Job drawing, mm, ordinate dimensions from the low corner. One solid piece. Give positions to 0.01 mm unless a question says otherwise; leave off trailing zeros. Write each loop counter-clockwise with the first axis right and the second up, starting at its lowest first coordinate (ties: lowest second). Pieces come first, ordered by that corner, then holes. Notation, with made-up numbers: (37.5, -37.5) -> (84.5, -37.5) arc R5 cw to (84.5, -33.5) -> close; hole circle Ø10 at (60, -25). An arc over 180 degrees is marked (long way). Put each result on its own line as item: value. Start each with the question number.
Item 1: Slice it at C-C, the plane x = 88.5. List the corners of the cut face in (y, z), plus the area to 3 significant figures.
Item 2: Slice it at D-D, the plane x = 28. List the corners of the cut face in (y, z).
Item 3: Flat gauge pins, fed straight in: pin 1 Ø12 at (x, y) = (73.5, 218.5) entering from -Z; pin 2 Ø1 at (x, z) = (108, 1.5) entering from +Y; pin 3 Ø1.9 at (x, z) = (35.5, 4) entering from +Y; pin 4 Ø1.5 at (x, z) = (106, 2.5) entering from +Y. Where does each tip first touch, or does it go through?
Item 4: Drill centre lines: line 1 along X through (y, z) = (66.5, 5) (1 decimal); line 2 along Y through (x, z) = (91.5, 5.75); line 3 along Y through (x, z) = (24.5, 4.25). Where is each one in solid material? Low to high.
Item 5: Slice it at A-A, the plane y = 142.5. Give the number of separate pieces and of enclosed holes in the cut face, plus the area to 3 significant figures.
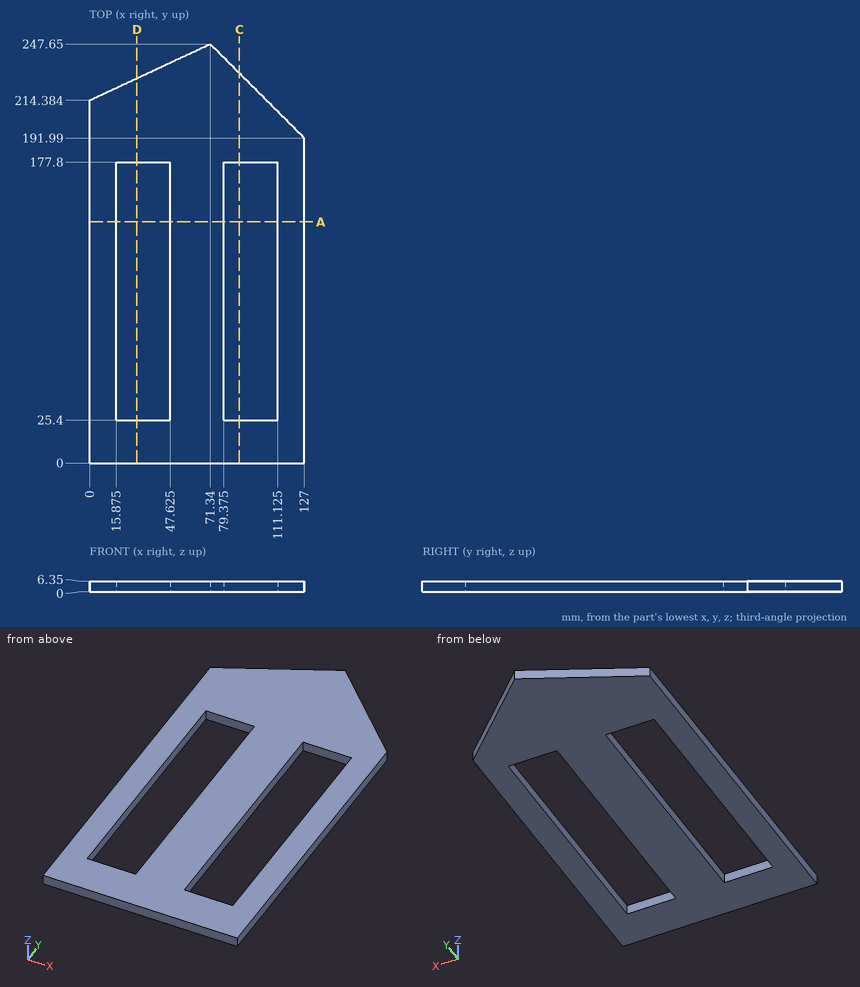
Values follow:
1. outline: (0, 0) -> (25.4, 0) -> (25.4, 6.35) -> (0, 6.35) -> close; (177.8, 0) -> (230.49, 0) -> (230.49, 6.35) -> (177.8, 6.35) -> close
1. area: 496 mm2
2. outline: (0, 0) -> (25.4, 0) -> (25.4, 6.35) -> (0, 6.35) -> close; (177.8, 0) -> (227.44, 0) -> (227.44, 6.35) -> (177.8, 6.35) -> close
3. pin 1: z = 0
3. pin 2: y = 211.49
3. pin 3: y = 231.38
3. pin 4: y = 213.74
4. line 1: 0 to 15.9, 47.6 to 79.4, 111.1 to 127
4. line 2: 0 to 25.4, 177.8 to 227.49
4. line 3: 0 to 25.4, 177.8 to 225.81
5. separate pieces: 3
5. enclosed holes: 0
5. area: 403 mm2
